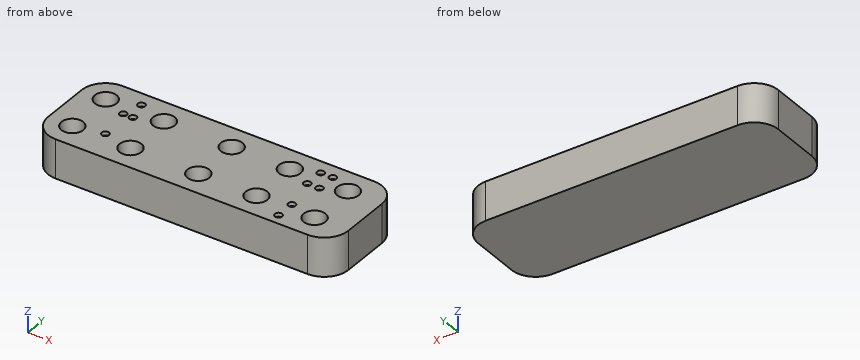
Autodesk Fusion 360 part; units mm, degrees
sketch "Sketch1" plane through (0, 0, 0) normal (0, 0, 1) x (1, 0, 0)
  circle A0 centre (-13, 0.815) radius 2.25
  circle A1 centre (-1, 0.815) radius 2.25
  circle A2 centre (13, 0.815) radius 2.25
  circle A3 centre (25, 0.815) radius 2.25
  circle A4 centre (37, 0.815) radius 2.25
  line L0 (-13, 0.815) -> (37, 0.815) construction
  circle A5 centre (-13, 10.815) radius 2.25
  circle A6 centre (-1, 10.815) radius 2.25
  circle A7 centre (13, 10.815) radius 2.25
  circle A8 centre (25, 10.815) radius 2.25
  circle A9 centre (37, 10.815) radius 2.25
  line L1 (-3, 4) -> (29, 4) construction
  line L2 (35.0527, 5.815) -> (-9.0686, 5.815) construction
  line L3 (-13, 10.815) -> (37, 10.815) construction
  line L4 (-13, 0.815) -> (37, 0.815) construction
  line L5 (-13, 0.815) -> (-13, 5.815) construction
  line L6 (-13, 5.815) -> (-13, 10.815) construction
  line L7 (-13, 5.815) -> (30, 5.815)
  line L8 (-13, 5.815) -> (-13, 15.815) construction
  line L9 (-13, 15.815) -> (39, 15.815)
  line L10 (-13, -4.185) -> (39, -4.185)
  line L11 (-13, 10.815) -> (-18, 10.815) construction
  arc A10 (-13, 15.815) -> (-18, 10.815) centre (-13, 10.815) ccw
  arc A11 (-18, 0.815) -> (-13, -4.185) centre (-13, 0.815) ccw
  line L12 (-18, 10.815) -> (-18, 0.815)
  line L13 (13, -4.185) -> (13, 15.815) construction
  arc A12 (44, 10.815) -> (39, 15.815) centre (39, 10.815) ccw
  line L14 (44, 10.815) -> (44, 0.815)
  arc A13 (39, -4.185) -> (44, 0.815) centre (39, 0.815) ccw
  point P0 (13, 4)
  dimension "d6" = 4.5
  dimension "d7" = 4.5
  dimension "d8" = 4.5
  dimension "d9" = 4.5
  dimension "d10" = 4.5
  dimension "d29" = 4.5
  dimension "d30" = 4.5
  dimension "d31" = 4.5
  dimension "d32" = 4.5
  dimension "d33" = 4.5
  dimension "d38" = 5
  dimension "d39" = 5
  dimension "d41" = 10
  dimension "M3_insert_taper_Ref" = -4
extrude "Extrude1" add sketch "Sketch1" along normal blind 8 contours A0 | A1 | A2 | A3 | A4 | A5 | A6 | A7 | A8 | A9 | L9 L10 A10 A11 L12 A12 L14 A13
extrude "Extrude4" cut sketch "Sketch1" against normal blind 5.8 draft -4 from surface at 8 contours A0 | A1 | A2 | A3 | A4 | A5 | A6 | A7 | A8 | A9
sketch "Sketch2" plane through (0, 0, 8) normal (0, 0, 1) x (-1, 0, 0)
  line L0 (11, 0) -> (3, 0) construction
  line L1 (7, 0) -> (7, -2) construction
  circle A0 centre (7, -2) radius 0.75
  line L2 (-27.5, 0) -> (-35.5, 0) construction
  line L3 (-35.5, 0) -> (-31.5, 0) construction
  line L4 (-31.5, 0) -> (-31.5, -2) construction
  circle A1 centre (-31.5, -2) radius 0.75
  circle A2 centre (-31.5, 2) radius 0.75
  line L5 (7, -10.815) -> (7, -12.815) construction
  line L6 (7, -12.815) -> (7, -10.815) construction
  line L7 (7, -10.815) -> (7, -8.815) construction
  line L8 (7, -8.815) -> (8, -8.815) construction
  line L9 (8, -8.815) -> (6, -8.815) construction
  circle A3 centre (8, -8.815) radius 0.75
  circle A4 centre (6, -8.815) radius 0.75
  circle A5 centre (7, -12.815) radius 0.75
  line L10 (-13, -10.815) -> (-13, -0.815) construction
  circle A6 centre (-32.5, -8.815) radius 0.75
  circle A7 centre (-30, -8.815) radius 0.75
  circle A8 centre (-32.5, -12.815) radius 0.75
  circle A9 centre (-30, -12.815) radius 0.75
  arc A10 (13, -15.815) -> (18, -10.815) centre (13, -10.815) ccw
  line L11 (18, -10.815) -> (18, -0.815)
  arc A11 (18, -0.815) -> (13, 4.185) centre (13, -0.815) ccw
  line L12 (13, 4.185) -> (-39, 4.185)
  arc A12 (-39, 4.185) -> (-44, -0.815) centre (-39, -0.815) ccw
  line L13 (-44, -0.815) -> (-44, -10.815)
  arc A13 (-44, -10.815) -> (-39, -15.815) centre (-39, -10.815) ccw
  line L14 (-39, -15.815) -> (13, -15.815)
  circle A14 centre (13, -0.815) radius 2.25
  circle A15 centre (-25, -0.815) radius 2.25
  circle A16 centre (-37, -0.815) radius 2.25
  circle A17 centre (-13, -10.815) radius 2.25
  circle A18 centre (1, -0.815) radius 2.25
  circle A19 centre (13, -10.815) radius 2.25
  circle A20 centre (-25, -10.815) radius 2.25
  circle A21 centre (-37, -10.815) radius 2.25
  circle A22 centre (1, -10.815) radius 2.25
  circle A23 centre (-13, -0.815) radius 2.25
  dimension "d14" = 1.5
  dimension "d15" = 2
  dimension "d16" = 1.5
  dimension "d21" = 1.5
  dimension "d22" = 1.5
  dimension "d23" = 1.5
  dimension "d35" = 1
  dimension "d36" = 1
extrude "Extrude2" cut sketch "Sketch2" against normal blind 0.8 contours A0 | A1 | A2 | A3 | A4 | A5 | A6 | A7 | A8 | A9
equation "d6 = d30"
equation "d7 = d30"
equation "d8 = d30"
equation "d9 = d30"
equation "d10 = d30"
equation "d16 = d14"
equation "d21 = d14"
equation "d22 = d14"
equation "d23 = d14"
equation "d27 = taper_angle"
equation "d29 = insert_diameter"
equation "d30 = d29"
equation "d31 = d30"
equation "d32 = d30"
equation "d33 = d30"
equation "M3_insert_dia_Ref = 4.5 mm"
equation "insert_diameter = M3_insert_dia_Ref"
equation "taper_angle = M3_insert_taper_Ref"
equation "insert_depth = M3_insert_depth_Ref"
CAD build for the part. Positions are in the model's coordinates, mm. Coordinates: 2 decimals unless noted, no trailing zeros. Order: outer loops, then holes, each group sorted by start corner. A loop starts at its lowest first (then second) coordinate and runs counter-clockwise, first axis right, second up. Notation, with made-up numbers: (88.25, -30.5) -> (102.25, -30.5) arc R21 cw to (102.25, -21.5) -> close; hole circle Ø4 at (63.25, 88.5). An arc over 180 degrees is marked (long way). Answer in a Markdown table with one row per item.
1) Band-saw the part on C-C (y = -2). List the corners of the cut face in (x, z), and give its area (3 significant figures).
Check values:
| item | result |
|---|---|
| outline | (-17.13, 0) -> (43.13, 0) -> (43.13, 8) -> (32.25, 8) -> (32.25, 7.2) -> (30.75, 7.2) -> (30.75, 8) -> (-17.13, 8) -> close |
| area | 481 mm2 |
2) Band-saw the part on D-D (z = 1). List the corners of the cut face in (x, y) (3 decimals), and give its area (3 significant figures).
Check values:
| item | result |
|---|---|
| outline | (-18, 0.815) arc R5 ccw to (-13, -4.185) -> (39, -4.185) arc R5 ccw to (44, 0.815) -> (44, 10.815) arc R5 ccw to (39, 15.815) -> (-13, 15.815) arc R5 ccw to (-18, 10.815) -> close |
| area | 1,220 mm2 |
3) Flat gauge pins, fed straight in: P1, Ø0.8, axis at x = 31.5, y = 2, coming from the +Z side; P2, Ø4, axis at y = 13.5, z = 7, coming from the -X side; P3, Ø1.8, axis at x = 13.5, y = 1.5, coming from the +Z side. Where does each tip first touch, or does it go through?
Check values:
| item | result |
|---|---|
| P1 | z = 7.2 |
| P2 | x = -17.95 |
| P3 | z = 2.2 |
4) Band-saw the part on A-A (z = 5.5). Give the number of separate pieces and of enclosed holes in the cut face, and give its area (3 significant figures).
Check values:
| item | result |
|---|---|
| separate pieces | 1 |
| enclosed holes | 10 |
| area | 1,080 mm2 |
5) Band-saw the part on B-B (x = 37). List the corners of the cut face in (y, z) (3 decimals), and give its area (3 significant figures).
Check values:
| item | result |
|---|---|
| outline | (-4.185, 0) -> (15.815, 0) -> (15.815, 8) -> (13.065, 8) -> (12.659, 2.2) -> (8.971, 2.2) -> (8.565, 8) -> (3.065, 8) -> (2.659, 2.2) -> (-1.029, 2.2) -> (-1.435, 8) -> (-4.185, 8) -> close |
| area | 113 mm2 |
6) Drill centre lines: line 1 (Y direction, x = 30, z = 7.8) (3 decimals); line 2 (Y direction, x = 31.5, z = 7.4) (3 decimals); line 3 (X direction, y = 10.25, z = 3.25). Where is each one in solid material? Low to high.
Check values:
| item | result |
|---|---|
| line 1 | -4.185 to 8.065, 9.565 to 12.065, 13.565 to 15.815 |
| line 2 | -4.185 to -2.75, -1.25 to 1.25, 2.75 to 15.815 |
| line 3 | -18 to -14.83, -11.17 to -2.83, 0.83 to 11.17, 14.83 to 23.17, 26.83 to 35.17, 38.83 to 44 |
